```python
from build123d import *

# Parameters (mm, degrees)
SKETCH1_W           = 15.875
SKETCH1_H           = 107.95
SKETCH1_R           = 2.159
BOSS_EXTRUDE1_DEPTH = 3.175


with BuildPart() as part:
    # Sketch1 → Boss-Extrude1 (new body)
    with BuildSketch(Plane.XY):
        with Locations((7.9375, 53.975)):
            Rectangle(SKETCH1_W, SKETCH1_H)
        with Locations((7.9375, 6.35)):
            Circle(SKETCH1_R, mode=Mode.SUBTRACT)
        with BuildLine():
            Line((10.1854, 101.6), (10.1854, 21.59))
            ThreePointArc((10.1854, 21.59), (7.9375, 19.3421), (5.6896, 21.59))
            Line((5.6896, 21.59), (5.6896, 101.6))
            ThreePointArc((5.6896, 101.6), (7.9375, 103.8479), (10.1854, 101.6))
        make_face(mode=Mode.SUBTRACT)
    extrude(amount=BOSS_EXTRUDE1_DEPTH)


solid = part.part
```
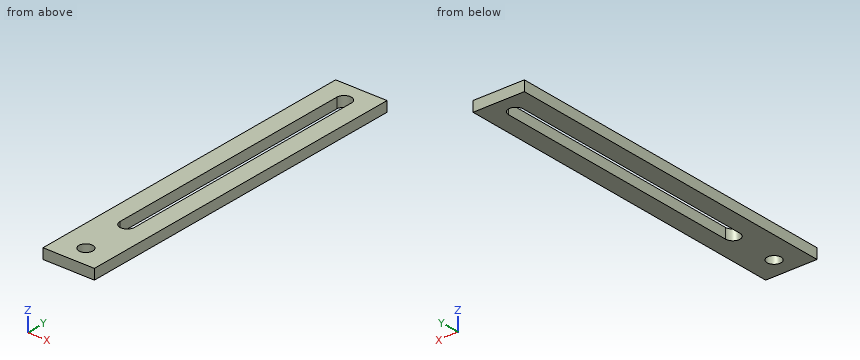
Build history of the part. All positions in model axes, mm. Coordinates: 2 decimals unless noted, no trailing zeros. Order: outer loops, then holes, each group sorted by start corner. A loop starts at its lowest first (then second) coordinate and runs counter-clockwise, first axis right, second up. Notation, with made-up numbers: (-7.5, 32.5) -> (33.5, 32.5) arc R9 ccw to (33.5, 42.5) -> close; hole circle Ø3 at (70.25, 85.5). An arc over 180 degrees is marked (long way). Answer in a Markdown table with one row per item. Add a question column.
Q1. Wall check: line 1 along Y through (x, z) = (8, 0.4); line 2 along X through (y, z) = (62, 0.9) (3 decimals); line 3 along Y through (x, z) = (6, 0.8). Give the ranges that are in metal, low to high. Write a range as [from, to].
Q2. Band-saw the part on A-A, the plane y = 6.35. List the corners of the cut face in (x, z) (1 decimal).
Q3. Band-saw the part on B-B, the plane z = 2.2. Give the number of separate pieces and of enclosed holes in the cut face, then the cut area to 3 significant figures.
Q4. Band-saw the part on C-C, the plane y = 47. List the corners of the cut face in (x, z) (3 decimals).
Answers follow:
| question | item | result |
|---|---|---|
| 1 | line 1 | [0, 4.19], [8.51, 19.34], [103.85, 107.95] |
| 1 | line 2 | [0, 5.69], [10.185, 15.875] |
| 1 | line 3 | [0, 5.4], [7.3, 20.45], [102.74, 107.95] |
| 2 | outline | (0, 0) -> (5.8, 0) -> (5.8, 3.2) -> (0, 3.2) -> close; (10.1, 0) -> (15.9, 0) -> (15.9, 3.2) -> (10.1, 3.2) -> close |
| 3 | separate pieces | 1 |
| 3 | enclosed holes | 2 |
| 3 | area | 1,320 mm^2 |
| 4 | outline | (0, 0) -> (5.69, 0) -> (5.69, 3.175) -> (0, 3.175) -> close; (10.185, 0) -> (15.875, 0) -> (15.875, 3.175) -> (10.185, 3.175) -> close |
